```python
from build123d import *

# Parameters (mm, degrees)
SKETCH1_R             = 1.6
BOSS_EXTRUDE2_DEPTH   = 5
BOSS_EXTRUDE2_2_DEPTH = 5
BOSS_EXTRUDE3_DEPTH   = 12
CUT_EXTRUDE1_DEPTH    = 2.3
CUT_EXTRUDE2_DEPTH    = 2.3
SKETCH4_R             = 1.6
CUT_EXTRUDE3_DEPTH    = 15
CUT_EXTRUDE4_DEPTH    = 2.3


with BuildPart() as part:
    # Sketch1 → Boss-Extrude2 (new body)
    with BuildSketch(Plane(origin=(0, 0, 0), x_dir=(1, 0, 0), z_dir=(0, 1, 0))):
        with BuildLine():
            ThreePointArc((-9.437293044, -4), (-10.25, 0), (-9.437293044, 4))
            Line((-9.437293044, 4), (-14.25, 4))
            ThreePointArc((-14.25, 4), (-18.25, 0), (-14.25, -4))
            Line((-14.25, -4), (-9.437293044, -4))
        make_face()
        with Locations(Location((-14.25, 0, 0), (0, 0, 270))):
            Circle(SKETCH1_R, mode=Mode.SUBTRACT)
    extrude(amount=BOSS_EXTRUDE2_DEPTH)



with BuildPart() as body_2:
    # Sketch1 → Boss-Extrude2 2 (new body)
    with BuildSketch(Plane(origin=(0, 0, 0), x_dir=(1, 0, 0), z_dir=(0, 1, 0))):
        with BuildLine():
            Line((42.25, 4), (37.437293044, 4))
            ThreePointArc((37.437293044, 4), (38.25, 0), (37.437293044, -4))
            Line((37.437293044, -4), (42.25, -4))
            ThreePointArc((42.25, -4), (46.25, 0), (42.25, 4))
        make_face()
        with Locations(Location((42.25, 0, 0), (0, 0, 270))):
            Circle(SKETCH1_R, mode=Mode.SUBTRACT)
    extrude(amount=BOSS_EXTRUDE2_2_DEPTH)


with BuildPart() as part_1:
    add(part.part)

    add(body_2.part)  # Boss-Extrude3 merges body 2
    # Sketch1_4 → Boss-Extrude3 (add)
    with BuildSketch(Plane(origin=(0, 0, 0), x_dir=(1, 0, 0), z_dir=(0, 1, 0))):
        with BuildLine():
            Line((9.5140033, 3.813953488), (18.4859967, 3.813953488))
            ThreePointArc((18.4859967, 3.813953488), (38.21590709, 0.835309718), (19.231923948, -5.308798579))
            Line((19.231923948, -5.308798579), (8.768076052, -5.308798579))
            ThreePointArc((8.768076052, -5.308798579), (-10.21590709, 0.835309718), (9.5140033, 3.813953488))
        make_face()
        with BuildLine():
            Line((9.195787079, 1), (18.804212921, 1))
            ThreePointArc((18.804212921, 1), (37.25, 0), (18.804212921, -1))
            Line((18.804212921, -1), (9.195787079, -1))
            ThreePointArc((9.195787079, -1), (-9.25, 0), (9.195787079, 1))
        make_face(mode=Mode.SUBTRACT)
    extrude(amount=BOSS_EXTRUDE3_DEPTH)

    # Sketch2 → Cut-Extrude1 (cut)
    with BuildSketch(Plane(origin=(0, 5, 0), x_dir=(1, 0, 0), z_dir=(0, 1, 0))):
        Polygon((-15.782040378, 2.814312044), (-17.453285913, 0.080370135), (-15.921245535, -2.733941909), (-12.717959622, -2.814312044), (-11.046714087, -0.080370135), (-12.578754465, 2.733941909), align=None)
    extrude(amount=-CUT_EXTRUDE1_DEPTH, mode=Mode.SUBTRACT)

    # Sketch3 → Cut-Extrude2 (cut)
    with BuildSketch(Plane(origin=(0, 5, 0), x_dir=(1, 0, 0), z_dir=(0, 1, 0))):
        Polygon((42.687046229, 3.180176713), (39.714409293, 1.968581494), (39.277363063, -1.211595219), (41.812953771, -3.180176713), (44.785590707, -1.968581494), (45.222636937, 1.211595219), align=None)
    extrude(amount=-CUT_EXTRUDE2_DEPTH, mode=Mode.SUBTRACT)

    # Sketch4 → Cut-Extrude3 (cut)
    with BuildSketch(Plane.XY.offset(5.308798579)):
        with Locations((14, 6)):
            Circle(SKETCH4_R)
    extrude(amount=-CUT_EXTRUDE3_DEPTH, mode=Mode.SUBTRACT)

    # Sketch7 → Cut-Extrude4 (cut)
    with BuildSketch(Plane.XY.offset(5.308798579)):
        Polygon((14.954593719, 9.05879892), (11.82829929, 8.356101871), (10.873705571, 5.297302951), (13.045406281, 2.94120108), (16.17170071, 3.643898129), (17.126294429, 6.702697049), align=None)
    extrude(amount=-CUT_EXTRUDE4_DEPTH, mode=Mode.SUBTRACT)


solid = part_1.part
```
The model under review builds one solid part; all positions refer to its coordinate system, in mm. A direction names the side the tool comes from. Give positions to 0.01 mm unless a question says otherwise; leave off trailing zeros. Write each loop counter-clockwise with the first axis right and the second up, starting at its lowest first coordinate (ties: lowest second). Pieces come first, ordered by that corner, then holes. Notation, with made-up numbers: (88, 59) - (110, 59) arc R25 ccw to (110, 91) - close; hole circle Ø8 at (-37, 32.25). An arc over 180 degrees is marked (long way). Answer in a Markdown table with one row per item. Add a question column.
1. We need section A-A on y = 10.75. Write out the cut boundary in (x, z), then the cut area to 3 significant figures.
2. Insertion check: P1, Ø1, axis at x = 36, y = 7.5, coming from the -Z side; P2, Ø2.5, axis at x = -11.5, y = 1.5, coming from the +Z side; P3, Ø4, axis at y = 6.5, z = -1.5, coming from the -X side. Each pin has a flat end and moves straight along its axis. Give the tip position at first contact, or say it passes through.
3. We need section D-D on x = 26. Write out the cut boundary in (y, z), then the cut area to 3 significant figures.
4. Wall thickness on line 1 along X through (y, z) = (1.7, 0); line 2 along Y through (x, z) = (14, 2.05); line 3 along X through (y, z) = (3.5, -5): over which ranges is each line inside the solid? List them lowest first. Write a range as [from, to].
5. Draft analysis for pull direction X (two halves, no side actions). For faces 1 (the flat face through (-12, 2, -4)), 2 (the cylindrical face through (46.25, 2.46, 0.09)), 3 (the flat face through (11.94, 4.14, 4.17)), state which applies: +X half, -X half, draft (parallel to the pull), parting line (faces both ways), or undercut.
6. We need section C-C on x = 14. Write out the cut boundary in (y, z), then the cut area to 3 significant figures.
7. Tool access review of faces 4 (the flat face through (44, 2.7, 1)), 5 (the flat face through (-12, 2, 4)), 6 (the flat face through (16.64, 5.15, 4.17)), 7 (the flat face through (12.9, 4.6, -3.814)): name each direction out of +Z, -Z, +X, -X, +Y, -Y from which nothing blocks a thin tool from reaching the whole face with its end or side.
8. We need section B-B on x = 0. Write out the cut boundary in (y, z), then the cut area to 3 significant figures.
Ans:
| question | item | result |
|---|---|---|
| 1 | outline | (8.77, 5.31) arc R10.25 ccw (long way) to (9.51, -3.81) - (18.49, -3.81) arc R10.25 ccw (long way) to (19.23, 5.31) - close; hole (9.2, -1) - (18.8, -1) arc R9.25 ccw (long way) to (18.8, 1) - (9.2, 1) arc R9.25 ccw (long way) to start |
| 1 | area | 179 mm^2 |
| 2 | P1 | stops at z = -6.99 |
| 2 | P2 | stops at z = 4 |
| 2 | P3 | stops at x = -18.25 |
| 3 | outline | (0, -10.05) - (12, -10.05) - (12, -9.03) - (0, -9.03) - close; (0, 9.03) - (12, 9.03) - (12, 10.05) - (0, 10.05) - close |
| 3 | area | 24.5 mm^2 |
| 4 | line 1 | x = [-18.25, -15.85], [-12.65, -9.25], [37.25, 40.65], [43.85, 46.25] |
| 4 | line 2 | y = [0, 4.4], [7.6, 12] |
| 4 | line 3 | x = [-8.95, -7.78], [7.78, 8.95], [19.05, 20.22], [35.78, 36.95] |
| 5 | face 1 | draft |
| 5 | face 2 | +X half |
| 5 | face 3 | undercut |
| 6 | outline | (0, -3.81) - (4.4, -3.81) - (4.4, -1) - (0, -1) - close; (0, 1) - (4.4, 1) - (4.4, 3.01) - (3.16, 3.01) - (3.16, 5.31) - (0, 5.31) - close; (7.6, -3.81) - (12, -3.81) - (12, -1) - (7.6, -1) - close; (7.6, 1) - (12, 1) - (12, 5.31) - (8.84, 5.31) - (8.84, 3.01) - (7.6, 3.01) - close |
| 6 | area | 57.0 mm^2 |
| 7 | face 4 | +Y |
| 7 | face 5 | +Z, -X, +Y, -Y |
| 7 | face 6 | +Z |
| 7 | face 7 | -Z, +Y, -Y |
| 8 | outline | (0, -10.25) - (12, -10.25) - (12, -9.25) - (0, -9.25) - close; (0, 9.25) - (12, 9.25) - (12, 10.25) - (0, 10.25) - close |
| 8 | area | 24.0 mm^2 |
